from build123d import *

# Parameters (mm, degrees)
BOSS_EXTRU_2_DEPTH         = 36.5
CONG_1_R                   = 0.5
ESQUISSE2_R                = 3.75
BOSS_EXTRU_3_DEPTH         = 2
ESQUISSE3_R                = 3
BOSS_EXTRU_4_DEPTH         = 1
ESQUISSE5_W                = 7.5
ESQUISSE5_H                = 37.315621328
ENL_V_MAT_EXTRU_2_DEPTH    = 5
ESQUISSE6_W                = 33
ESQUISSE6_H                = 22
BOSS_EXTRU_6_DEPTH         = 0.5
ESQUISSE7_W                = 22.000592026
ESQUISSE7_H                = 17.5
BOSS_EXTRU_7_DEPTH         = 0.5
ESQUISSE8_W                = 21.996306334
ESQUISSE8_H                = 17.5
BOSS_EXTRU_8_DEPTH         = 0.5
ESQUISSE9_W                = 5.5
ESQUISSE9_H                = 22
ENL_V_MAT_EXTRU_3_DEPTH    = 0.5
ESQUISSE10_R               = 2
ENL_V_MAT_EXTRU_4_DEPTH    = 10.5
ESQUISSE11_W               = 2.1
ESQUISSE11_H               = 7.00005
TROU_TARAUD_M51_AT_2_COUNT = 2
TROU_TARAUD_M51_AT_2_PITCH = 25.902595086


# Read off the part's stored shape, not the designer's step: Dôme1
with BuildPart() as part:
    # Esquisse1 → Boss.-Extru.2 (new body)
    with BuildSketch(Plane.XY):
        Polygon((-16.5, 0), (-16.5, 10.25), (-22.270485302, 10.25), (-24.856553081, 10.25), (-24.856553081, 12.366468473), (-24.25, 12.366468473), (-23.5, 14.775104227), (-23.5, 15.186461692), (-23, 15.684420728), (-25.5, 17), (-33, 17), (-33, 0), align=None)
        Polygon((-10.729514698, 10.25), (-16.5, 10.25), (-16.5, 0), (0, 0), (0, 17), (-7.5, 17), (-10, 15.684420728), (-9.5, 15.186461692), (-9.5, 14.775104227), (-8.75, 12.366468473), (-8.143446919, 12.366468473), (-8.143446919, 10.25), align=None)
    extrude(amount=BOSS_EXTRU_2_DEPTH)

    # Congé1
    cong_1_edges = [part.edges().sort_by_distance(p)[0] for p in [
        (-23.5, 15.186461692, 18.25),
        (-24.856553081, 10.25, 18.25),
        (-8.143446919, 10.25, 18.25),
        (-9.5, 15.186461692, 18.25),
    ]]
    fillet(cong_1_edges, radius=CONG_1_R)

    # Esquisse2 → Boss.-Extru.3 (add)
    with BuildSketch(Plane(origin=(0, 0, 0), x_dir=(-1, 0, 0), z_dir=(0, 0, -1))):
        with Locations(Location((16.5, 5.125, 0), (0, 0, 180))):
            Circle(ESQUISSE2_R)
    extrude(amount=BOSS_EXTRU_3_DEPTH)

    # Esquisse3 → Boss.-Extru.4 (add)
    with BuildSketch(Plane(origin=(0, 0, -2), x_dir=(-1, 0, 0), z_dir=(0, 0, -1))):
        with Locations((16.5, 5.125)):
            Circle(ESQUISSE3_R)
    extrude(amount=BOSS_EXTRU_4_DEPTH)

    # Dôme1 outline → Dôme1 (revolve)
    with BuildSketch(Plane(origin=(-16.5, 5.125, 0), x_dir=(1, 0, 0), z_dir=(0, -1, 0))):
        with BuildLine():
            Line((0, -2.999999997), (0, -6))
            ThreePointArc((0, -6), (2.121320345, -5.121320342), (3, -2.999999997))
            Line((3, -2.999999997), (0, -2.999999997))
        make_face()
    revolve(axis=Axis((-16.5, 5.125, 0), (0, 0, 1)))

    # Esquisse5 → Enlèv. mat.-Extru.2 (cut)
    with BuildSketch(Plane(origin=(0, 17, 0), x_dir=(1, 0, 0), z_dir=(0, 1, 0))):
        with Locations((-12.75, -18.657810664)):
            Rectangle(ESQUISSE5_W, ESQUISSE5_H)
        with Locations((-20.25, -18.657810664)):
            Rectangle(ESQUISSE5_W, ESQUISSE5_H)
    extrude(amount=-ENL_V_MAT_EXTRU_2_DEPTH, mode=Mode.SUBTRACT)

    # Esquisse6 → Boss.-Extru.6 (add)
    with BuildSketch(Plane(origin=(0, 0, 0), x_dir=(-1, 0, 0), z_dir=(0, -1, 0))):
        with Locations((16.5, -18.25)):
            Rectangle(ESQUISSE6_W, ESQUISSE6_H)
    extrude(amount=BOSS_EXTRU_6_DEPTH)

    # Esquisse7 → Boss.-Extru.7 (add)
    with BuildSketch(Plane(origin=(0, 0, 0), x_dir=(0, 0, -1), z_dir=(1, 0, 0))):
        with Locations((-18.250296013, 8.25)):
            Rectangle(ESQUISSE7_W, ESQUISSE7_H)
    extrude(amount=BOSS_EXTRU_7_DEPTH)

    # Esquisse8 → Boss.-Extru.8 (add)
    with BuildSketch(Plane.ZY.offset(33)):
        with Locations((18.251846833, 8.25)):
            Rectangle(ESQUISSE8_W, ESQUISSE8_H)
    extrude(amount=BOSS_EXTRU_8_DEPTH)

    # Esquisse9 → Enlèv. mat.-Extru.3 (cut)
    with BuildSketch(Plane(origin=(0, -0.5, 0), x_dir=(-1, 0, 0), z_dir=(0, -1, 0))):
        with Locations((14, -18.25)):
            Rectangle(ESQUISSE9_W, ESQUISSE9_H)
        with Locations((19.5, -18.25)):
            Rectangle(ESQUISSE9_W, ESQUISSE9_H)
    extrude(amount=-ENL_V_MAT_EXTRU_3_DEPTH, mode=Mode.SUBTRACT)

    # Esquisse10 → Enlèv. mat.-Extru.4 (cut)
    with BuildSketch(Plane.XZ.offset(0.5)):
        with Locations(Location((-3.5, 18.250296013, 0), (0, 0, 270))):
            Circle(ESQUISSE10_R)
        with Locations(Location((-29.5, 18.250296013, 0), (0, 0, 270))):
            Circle(ESQUISSE10_R)
    extrude(amount=-ENL_V_MAT_EXTRU_4_DEPTH, mode=Mode.SUBTRACT)

    # Esquisse11 → Trou taraudé M51 (revolve, cut)
    with BuildSketch(Plane(origin=(-29.402494858, 10, 18.178238283), x_dir=(0, 0, -1), z_dir=(1, 0, 0))):
        with Locations((1.05, 3.500025)):
            Rectangle(ESQUISSE11_W, ESQUISSE11_H)
    trou_taraud_m51 = revolve(axis=Axis((-29.402494858, 3.65, 18.178238283), (0, 1, 0)), mode=Mode.SUBTRACT)

    # Trou taraudé M51 at 2: Trou taraudé M51 ×2
    with Locations(*[Vector(0.9999961305838194, 0, 0.002781873000113731) * (i * TROU_TARAUD_M51_AT_2_PITCH) for i in range(1, TROU_TARAUD_M51_AT_2_COUNT)]):
        add(trou_taraud_m51, mode=Mode.SUBTRACT)


solid = part.part
Here's how the part is built. I have some questions about the finished solid (model axes, mm). A direction names the side the tool comes from. Round coordinates to 2 decimals unless told otherwise and drop trailing zeros. Loops run counter-clockwise (first coordinate to the right, second up) from the corner with the lowest first, then second, coordinate; pieces in that order, holes last. Notation, with made-up numbers: (80.5, 82.25) - (123.5, 82.25) arc R9 ccw to (123.5, 96.25) - close; hole circle Ø6 at (80.5, 38). An arc over 180 degrees is marked (long way). One line per question, with ' | ' between items. Start each with the question number.
Q1. I want a section at C-C (x = -7). Write out the boundary of the cut face in (y, z), then the cut area to 4 significant figures.
Q2. For faces 1 (the flat face through (-8.143, 12, 18)), 2 (the cylindrical face through (-4.92, 13.55, 19.8)), 3 (the flat face through (-24, 15, 19)), 4 (the flat face through (-33, 8, 4)), which set-ups out of +Z, -Z, +X, -X, +Y, -Y let a thin tool reach every point of the face, with its end or its side?
Q3. Will these pins go through, and if not, where does the flat tip stop? pin 1 (3.5 mm diameter, centred on y = 10, z = 31.5, fed in from +X); pin 2 (1 mm diameter, centred on x = -21.5, y = 7.5, fed in from -Z); pin 3 (4 mm diameter, centred on x = -11.5, z = 16, fed in from +Y).
Q4. We'd pull the mould along Y, two halves only. Please class faces 5 (the flat face through (-24.74, 16.6, 17.99)), 6 (the flat face through (-33, 9, 33)), 7 (the flat face through (-24.857, 12, 18)): +Y half, -Y half, draft (parallel to the pull), parting line (faces both ways), or undercut.
Q5. I want a section at B-B (y = 11.25). Write out the boundary of the cut face in (x, z), then the cut area to 3 significant figures.
Q6. I want a section at D-D (z = 1). Write out the boundary of the cut face in (x, y).
Q7. I want a section at A-A (x = -3.5). Write out the boundary of the cut face in (y, z), then the cut area to 3 significant figures.
Q8. Please list where these lines run through material, in increasing order: line 1 (X direction, y = 12, z = 34.5); line 2 (Z direction, x = -29.5, y = 11.25); line 3 (Z direction, x = -3, y = 14.5). Write a range as [from, to].
Response values:
1) outline: (-0.5, 7.25) - (0, 7.25) - (0, 0) - (17, 0) - (17, 36.5) - (0, 36.5) - (0, 29.25) - (-0.5, 29.25) - close | area: 631.5 mm²
2) face 1: +Z, -Z | face 2: +Y | face 3: +Z, -Z, +Y | face 4: -Z, -X, +Y, -Y
3) pin 1: stops at x = 0 | pin 2: stops at z = 0 | pin 3: stops at y = 10.25
4) face 5: +Y half | face 6: draft | face 7: undercut
5) outline: (-33.5, 7.25) - (-33, 7.25) - (-33, 0) - (-24.86, 0) - (-24.86, 36.5) - (-33, 36.5) - (-33, 29.25) - (-33.5, 29.25) - close; (-8.14, 0) - (0, 0) - (0, 7.25) - (0.5, 7.25) - (0.5, 29.25) - (0, 29.25) - (0, 36.5) - (-8.14, 36.5) - close; hole circle Ø4.2 at (-29.4, 18.18); hole circle Ø4.2 at (-3.5, 18.25) | area: 589 mm²
6) outline: (-33, 0) - (0, 0) - (0, 17) - (-7.5, 17) - (-9, 16.21) - (-9, 13.17) - (-8.75, 12.37) - (-8.14, 12.37) - (-8.14, 10.75) arc R0.5 cw to (-8.64, 10.25) - (-24.36, 10.25) arc R0.5 cw to (-24.86, 10.75) - (-24.86, 12.37) - (-24.25, 12.37) - (-24, 13.17) - (-24, 16.21) - (-25.5, 17) - (-33, 17) - close
7) outline: (-0.5, 7.25) - (0, 7.25) - (0, 0) - (17, 0) - (17, 16.15) - (10, 16.15) - (10, 16.25) - (-0.5, 16.25) - close; (-0.5, 20.25) - (10, 20.25) - (10, 20.35) - (17, 20.35) - (17, 36.5) - (0, 36.5) - (0, 29.25) - (-0.5, 29.25) - close | area: 560 mm²
8) line 1: x = [-33, -24.86], [-8.14, 0] | line 2: z = [0, 16.08], [20.28, 36.5] | line 3: z = [0, 16.21], [20.29, 36.5]
